```python
from build123d import *

# Parameters (mm, degrees)
SKETCH_1_W            = 81.9
SKETCH_1_H            = 67.9
EXTRUDE_1_DEPTH       = 10
SKETCH_2_W            = 60.5
SKETCH_2_H            = 60.5
CUT_EXTRUDE_1_DEPTH   = 8.5
CUT_EXTRUDE_4_REACH   = 91.242
M2_5X0_451_AT_2_COUNT = 2
M2_5X0_451_AT_2_PITCH = 67.264213562
CUT_EXTRUDE_5_REACH   = 81.921
CUT_EXTRUDE_6_REACH   = 81.129
CUT_EXTRUDE_7_REACH   = 54.949


with BuildPart() as part:
    # Эскиз1 → Бобышка-Вытянуть1 (new body)
    with BuildSketch(Plane.XY):
        Rectangle(SKETCH_1_W, SKETCH_1_H)
    extrude(amount=-EXTRUDE_1_DEPTH)

    # Эскиз2 → Вырез-Вытянуть1 (cut)
    with BuildSketch(Plane(origin=(0, 0, -10), x_dir=(-1, 0, 0), z_dir=(0, 0, -1))):
        Rectangle(SKETCH_2_W, SKETCH_2_H)
    extrude(amount=-CUT_EXTRUDE_1_DEPTH, mode=Mode.SUBTRACT)

    # Эскиз4 → Вырез-Вытянуть4 (cut, up to next)
    with BuildSketch(Plane(origin=(0, -33.95, -40.95), x_dir=(1, 0, 0), z_dir=(0, 1, 0)), mode=Mode.PRIVATE) as cut_extrude_4_sk1:
        with BuildLine():
            Line((39.383021279, -39.383021279), (40.95, -40.95))
            Line((40.95, -40.95), (35.6, -40.95))
            ThreePointArc((35.6, -40.95), (37.647356363, -40.542755499), (39.383021279, -39.383021279))
        make_face()
    cut_extrude_4_tool1 = extrude(cut_extrude_4_sk1.sketch, amount=CUT_EXTRUDE_4_REACH, mode=Mode.PRIVATE) & part.part
    # Эскиз4 → Вырез-Вытянуть4 (cut, up to next)
    with BuildSketch(Plane(origin=(0, -33.95, -40.95), x_dir=(1, 0, 0), z_dir=(0, 1, 0)), mode=Mode.PRIVATE) as cut_extrude_4_sk2:
        with BuildLine():
            Line((-40.95, -40.95), (-35.6, -40.95))
            ThreePointArc((-35.6, -40.95), (-37.647356363, -40.542755499), (-39.383021279, -39.383021279))
            Line((-39.383021279, -39.383021279), (-40.95, -40.95))
        make_face()
    cut_extrude_4_tool2 = extrude(cut_extrude_4_sk2.sketch, amount=CUT_EXTRUDE_4_REACH, mode=Mode.PRIVATE) & part.part
    add(cut_extrude_4_tool1.solids().sort_by_distance((39.042099, -33.95, -0.482136))[0], mode=Mode.SUBTRACT)
    add(cut_extrude_4_tool2.solids().sort_by_distance((-39.042099, -33.95, -0.482136))[0], mode=Mode.SUBTRACT)

    # Эскиз8 → Отверстие обработанное метчиком M2.5x0.451 (revolve, cut)
    with BuildSketch(Plane(origin=(33.632106781, 33.95, -3.382106781), x_dir=(0, 0, 1), z_dir=(1, 0, 0))):
        Polygon((0, 0), (0, 5.615882135), (1.025, 5), (1.025, 0), align=None)
    m2_5x0_451 = revolve(axis=Axis((33.632106781, 40.3, -3.382106781), (0, -1, 0)), mode=Mode.SUBTRACT)

    # Отверстие обработанное метчиком M2.5x0.451 at 2: Отверстие обработанное метчиком M2.5x0.451 ×2
    with Locations(*[(-i * M2_5X0_451_AT_2_PITCH, 0, 0) for i in range(1, M2_5X0_451_AT_2_COUNT)]):
        add(m2_5x0_451, mode=Mode.SUBTRACT)

    # Зеркальное отражение1: Отверстие обработанное метчиком M2.5x0.451 across plane
    add(m2_5x0_451.mirror(Plane.ZX), mode=Mode.SUBTRACT)

    # Зеркальное отражение1 copy 1 sketch → Зеркальное отражение1 copy 1 (revolve, cut)
    with BuildSketch(Plane(origin=(-33.632106781, -33.95, -3.382106781), x_dir=(0, 0, 1), z_dir=(1, 0, 0))):
        Polygon((0, 0), (0, -5.615882135), (1.025, -5), (1.025, 0), align=None)
    revolve(axis=Axis((-33.632106781, -40.3, -3.382106781), (0, -1, 0)), mode=Mode.SUBTRACT)

    # Эскиз3 → Вырез-Вытянуть5 (cut, up to next)
    with BuildSketch(Plane(origin=(0, 33.95, 0), x_dir=(1, 0, 0), z_dir=(0, 1, 0)), mode=Mode.PRIVATE) as cut_extrude_5_sk1:
        Polygon((30.95, 10), (40.95, 0), (40.95, 10), align=None)
    cut_extrude_5_tool1 = extrude(cut_extrude_5_sk1.sketch, amount=-CUT_EXTRUDE_5_REACH, mode=Mode.PRIVATE) & part.part
    # Эскиз3 → Вырез-Вытянуть5 (cut, up to next)
    with BuildSketch(Plane(origin=(0, 33.95, 0), x_dir=(1, 0, 0), z_dir=(0, 1, 0)), mode=Mode.PRIVATE) as cut_extrude_5_sk2:
        Polygon((-30.95, 10), (-40.95, 10), (-40.95, 0), align=None)
    cut_extrude_5_tool2 = extrude(cut_extrude_5_sk2.sketch, amount=-CUT_EXTRUDE_5_REACH, mode=Mode.PRIVATE) & part.part
    add(cut_extrude_5_tool1.solids().sort_by_distance((37.616667, 33.95, -6.666667))[0], mode=Mode.SUBTRACT)
    add(cut_extrude_5_tool2.solids().sort_by_distance((-37.616667, 33.95, -6.666667))[0], mode=Mode.SUBTRACT)

    # Эскиз10 → Вырез-Вытянуть6 (cut, up to next)
    with BuildSketch(Plane(origin=(0, 33.95, 0), x_dir=(1, 0, 0), z_dir=(0, 1, 0)), mode=Mode.PRIVATE) as cut_extrude_6_sk1:
        Polygon((24.022188141, 3.002183714), (12.522188141, 3.002183714), (12.522188141, 7.45), (-17.477811859, 7.45), (-17.477811859, 10), (12.522188141, 10), (24.022188141, 10), align=None)
    cut_extrude_6_tool1 = extrude(cut_extrude_6_sk1.sketch, amount=-CUT_EXTRUDE_6_REACH, mode=Mode.PRIVATE) & part.part
    add(cut_extrude_6_tool1.solids().sort_by_distance((8.159902, 33.95, -7.584889))[0], mode=Mode.SUBTRACT)

    # Эскиз11 → Вырез-Вытянуть7 (cut, up to next)
    with BuildSketch(Plane.XY, mode=Mode.PRIVATE) as cut_extrude_7_sk1:
        with BuildLine():
            Line((14.437188141, 33.571201289), (14.437188141, 32.976592334))
            add(Edge.make_bspline(
                [(14.437188141, 32.976592334), (14.451126829, 32.828049776), (14.506397384, 32.534626701), (14.763436949, 32.126248808), (15.171814842, 31.869209242), (15.465237917, 31.813938687), (15.613780476, 31.8)],
                knots=[-0.018208692, -0.018208692, -0.018208692, -0.018208692, 0.240895654, 0.5, 0.759104346, 1.018208692, 1.018208692, 1.018208692, 1.018208692], degree=3))
            Line((15.613780476, 31.8), (20.930595807, 31.8))
            add(Edge.make_bspline(
                [(20.930595807, 31.8), (21.079138366, 31.813938687), (21.37256144, 31.869209242), (21.780939333, 32.126248808), (22.037978899, 32.534626701), (22.093249454, 32.828049776), (22.107188141, 32.976592334)],
                knots=[-0.018208692, -0.018208692, -0.018208692, -0.018208692, 0.240895654, 0.5, 0.759104346, 1.018208692, 1.018208692, 1.018208692, 1.018208692], degree=3))
            Line((22.107188141, 32.976592334), (22.107188141, 33.591493881))
            add(Edge.make_bspline(
                [(22.107188141, 33.591493881), (22.535068025, 33.877662587), (22.962947908, 34.163831294), (23.390827792, 34.45)],
                knots=[1.333301569, 1.333301569, 1.333301569, 1.333301569, 6.343818338, 6.343818338, 6.343818338, 6.343818338], degree=3))
            Line((23.390827792, 34.45), (13.216758216, 34.45))
            add(Edge.make_bspline(
                [(13.216758216, 34.45), (13.623568191, 34.157067096), (14.030378166, 33.864134193), (14.437188141, 33.571201289)],
                knots=[1.296985877, 1.296985877, 1.296985877, 1.296985877, 5.968647001, 5.968647001, 5.968647001, 5.968647001], degree=3))
        make_face()
    cut_extrude_7_tool1 = extrude(cut_extrude_7_sk1.sketch, amount=-CUT_EXTRUDE_7_REACH, mode=Mode.PRIVATE) & part.part
    add(cut_extrude_7_tool1.solids().sort_by_distance((18.275758, 33.211289, 0))[0], mode=Mode.SUBTRACT)


solid = part.part
```
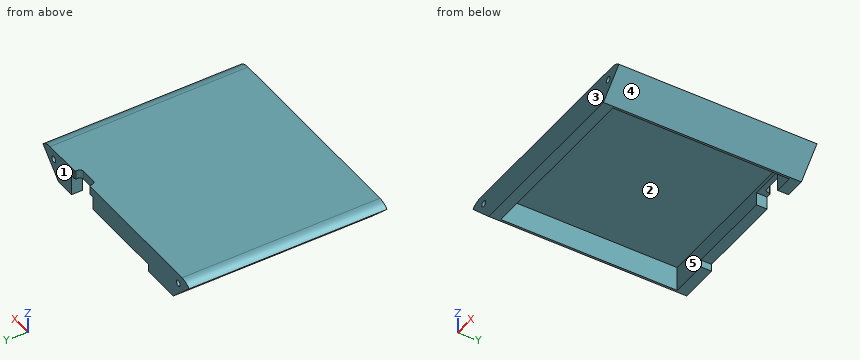
Geometry: final body of the model. Coordinates: model frame, mm. Face numbers are marked on the shaded views. A direction names the side the tool comes from. Give positions to 0.01 mm unless a question says otherwise; leave off trailing zeros. Loops run counter-clockwise (first coordinate to the right, second up) from the corner with the lowest first, then second, coordinate; pieces in that order, holes last. Notation, with made-up numbers: (-39, 52) -> (0, 52) arc R25 ccw to (0, 91) -> close; hole circle Ø2 at (-2.75, -37.75). An arc over 180 degrees is marked (long way). Use CSV: the item, a comma, the result in double quotes.
(1) Cut plane D-D (x = 27). Output: boundary loops of the cut face in (y, z), plus the area to 3 significant figures.
From the geometry:
outline,"(-33.95, -10) -> (-30.25, -10) -> (-30.25, -1.5) -> (30.25, -1.5) -> (30.25, -10) -> (33.95, -10) -> (33.95, 0) -> (-33.95, 0) -> close"
area,"165 mm^2"
(2) First-contact query: P1, Ø1.8, axis at x = 33.63, z = -3.38, coming from the -Y side; P2, Ø1.5, axis at x = 13, y = 27, coming from the -Z side; P3, Ø1.6, axis at x = -33.63, z = -3.38, coming from the -Y side. Flat tips, straight axial feed; report the tip coordinate or a pass-through.
From the geometry:
P1,"y = -28.88"
P2,"z = -1.5"
P3,"y = -28.82"
(3) Access query for the marked faces 1 and 2. Directions: +Z, -Z, +X, -X, +Y, -Y. A direction counts if a zero-diameter tool reaches every point of the face in a straight line with its end or side. Return the directions, or none.
From the geometry:
face 1,"+Z, -Z, +X, -X, +Y"
face 2,"-Z"
(4) Cut plane B-B (x = 3). Output: boundary loops of the cut face in (y, z), plus the area to 3 significant figures.
From the geometry:
outline,"(-33.95, -10) -> (-30.25, -10) -> (-30.25, -1.5) -> (30.25, -1.5) -> (30.25, -7.45) -> (33.95, -7.45) -> (33.95, 0) -> (-33.95, 0) -> close"
area,"155 mm^2"
(5) Ray query, line 1 along Y through (x, z) = (2, -5.5); line 2 along Y through (x, z) = (17, -4.5). Return the intervals inside material, ascending. Write a range as [from, to].
From the geometry:
line 1,"[-33.95, -30.25], [30.25, 33.95]"
line 2,"[-33.95, -30.25]"
(6) Pull-direction query (X, two-part tool) for the marked faces 3, 4 and 5; classes: released by +X, released by -X, zero draft, split by the parting line, or undercut.
From the geometry:
face 3,"zero draft"
face 4,"released by +X"
face 5,"undercut"
(7) Cut plane A-A (z = -8.5). Output: boundary loops of the cut face in (x, y).
From the geometry:
outline,"(-32.45, -33.95) -> (32.45, -33.95) -> (32.45, 33.95) -> (24.02, 33.95) -> (24.02, 30.25) -> (30.25, 30.25) -> (30.25, -30.25) -> (-30.25, -30.25) -> (-30.25, 30.25) -> (-17.48, 30.25) -> (-17.48, 33.95) -> (-32.45, 33.95) -> close"
(8) Cut plane C-C (y = -26.5). Output: boundary loops of the cut face in (x, z), plus the area to 3 significant figures.
From the geometry:
outline,"(-39.38, -1.57) -> (-30.95, -10) -> (-30.25, -10) -> (-30.25, -1.5) -> (30.25, -1.5) -> (30.25, -10) -> (30.95, -10) -> (39.38, -1.57) arc R5.35 ccw to (35.6, 0) -> (-35.6, 0) arc R5.35 ccw to start"
area,"199 mm^2"
